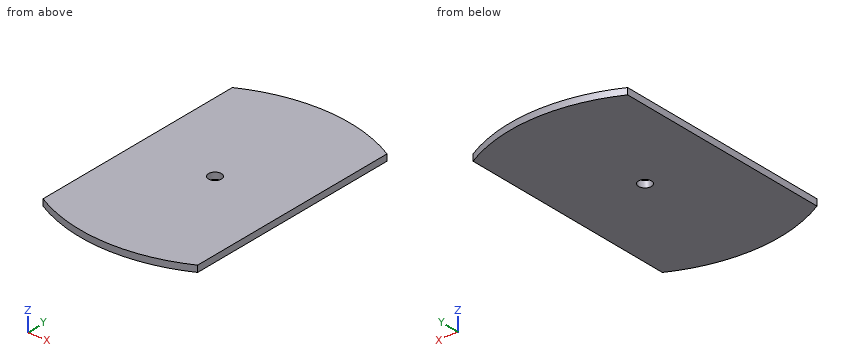
Autodesk Fusion 360 part; units mm, degrees
sketch "Esquisse1" plane through (0, 0, 0) normal (0, 0, 1) x (1, 0, 0)
  line L0 (60, -86) -> (-60, -86)
  line L1 (-60, -86) -> (-60, 86)
  line L2 (-60, 86) -> (60, 86)
  line L3 (60, 86) -> (60, -86)
  line L4 (60, -86) -> (-60, 86) construction
  line L5 (-60, -86) -> (60, 86) construction
  dimension "d1" = 120
  dimension "d2" = 172
sketch "Esquisse2" plane through (0, 0, 0) normal (0, 0, 1) x (1, 0, 0)
  line L0 (0, -86) -> (0, -101)
  line L1 (0, 86) -> (0, 101)
  line L2 (60, -86) -> (-60, -86)
  line L3 (-60, -86) -> (-60, -116)
  line L4 (-60, -116) -> (60, -116)
  line L5 (60, -116) -> (60, -86)
  line L6 (60, -86) -> (-60, -116) construction
  line L7 (-60, -86) -> (60, -116) construction
  line L8 (-60, 86) -> (60, 86)
  line L9 (60, 86) -> (60, 116)
  line L10 (60, 116) -> (-60, 116)
  line L11 (-60, 116) -> (-60, 86)
  line L12 (-60, 86) -> (60, 116) construction
  line L13 (60, 86) -> (-60, 116) construction
  arc A0 (60, 86) -> (-60, 86) centre (0, -26.5) ccw
  arc A1 (-60, -86) -> (60, -86) centre (0, 26.5) ccw
  point P0 (0, -101)
  point P1 (0, 101)
  dimension "d3" = 15
  dimension "d4" = 15
extrude "Extrusion1" add sketch "Esquisse1" sketch "Esquisse2" along normal blind 10 of sketch 2 contours L0 L2 A1 | L0 L2 A1 | L1 L8 A0 | L1 L8 A0
sketch "Esquisse3" plane through (0, 0, 10) normal (0, 0, 1) x (-1, 0, 0)
  line L0 (60, -86) -> (60, 86)
  arc A0 (60, 86) -> (-60, 86) centre (0, -26.5) ccw
  line L1 (-60, 86) -> (-60, -86)
  arc A1 (-60, -86) -> (60, -86) centre (0, 26.5) ccw
  line L2 (60, 86) -> (-60, 86)
  line L3 (60, -86) -> (-60, -86)
  line L4 (-60, 86) -> (-60, 70)
  line L5 (-60, 70) -> (-60, 48)
  line L6 (-60, 48) -> (-60, -48)
  line L7 (-60, -48) -> (-60, -70)
  line L8 (60, 86) -> (60, 70)
  line L9 (60, 70) -> (60, 48)
  line L10 (60, 48) -> (60, -48)
  line L11 (60, -48) -> (60, -70)
  line L12 (60, 70) -> (36, 70)
  line L13 (36, 70) -> (36, 48)
  line L14 (36, 48) -> (60, 48)
  line L15 (60, -70) -> (36, -70)
  line L16 (36, -70) -> (36, -48)
  line L17 (36, -48) -> (60, -48)
  line L18 (-60, -70) -> (-36, -70)
  line L19 (-36, -70) -> (-36, -48)
  line L20 (-36, -48) -> (-60, -48)
  line L21 (-60, 70) -> (-36, 70)
  line L22 (-36, 70) -> (-36, 48)
  line L23 (-60, 48) -> (-36, 48)
  dimension "d7" = 16
  dimension "d8" = 22
  dimension "d9" = 96
  dimension "d10" = 22
  dimension "d11" = 16
  dimension "d12" = 22
  dimension "d13" = 96
  dimension "d14" = 22
  dimension "d15" = 24
  dimension "d16" = 24
  dimension "d17" = 22
sketch "Esquisse4" plane through (0, 0, 10) normal (0, 0, 1) x (-1, 0, 0)
  line L0 (-60, -86) -> (-17, -86)
  line L1 (-17, -86) -> (17, -86)
  line L2 (17, -86) -> (17, -70)
  line L3 (17, -70) -> (-17, -70)
  line L4 (-17, -70) -> (-17, -86)
  dimension "d18" = 43
  dimension "d19" = 34
extrude "Extrusion2" cut sketch "Esquisse3" against normal blind 5
extrude "Extrusion3" cut sketch "Esquisse4" along normal blind 0 and the other way blind 25
sketch "Esquisse5" plane through (0, 0, 5) normal (0, 0, 1) x (-1, 0, 0)
  line L0 (17, -86) -> (-17, -86)
  line L1 (-17, -86) -> (-17, -70)
  line L2 (-17, -70) -> (17, -70)
  line L3 (17, -70) -> (17, -86)
  arc A0 (60, 86) -> (-60, 86) centre (0, -26.5) ccw
  line L4 (-60, 86) -> (-60, -86)
  arc A1 (-60, -86) -> (60, -86) centre (0, 26.5) ccw
  line L5 (60, -86) -> (60, 86)
  line L6 (-60, -86) -> (60, -86)
  line L7 (-60, 86) -> (60, 86)
  line L8 (-60, -86) -> (-60, -70)
  line L9 (-60, -70) -> (-60, -48)
  line L10 (-60, -48) -> (-60, 48)
  line L11 (-60, 48) -> (-60, 70)
  line L12 (-60, -70) -> (-36, -70)
  line L13 (-36, -70) -> (-36, -48)
  line L14 (-36, -48) -> (-60, -48)
  line L15 (-60, 70) -> (-36, 70)
  line L16 (-60, 48) -> (-36, 48)
  line L17 (-36, 48) -> (-36, 70)
  line L18 (60, -70) -> (36, -70)
  line L19 (36, -70) -> (36, -48)
  line L20 (36, -48) -> (60, -48)
  line L21 (60, 48) -> (36, 48)
  line L22 (36, 48) -> (36, 70)
  line L23 (36, 70) -> (60, 70)
  dimension "d27" = 16
  dimension "d28" = 22
  dimension "d29" = 96
  dimension "d30" = 22
  dimension "d31" = 24
  dimension "d32" = 24
sketch "Esquisse6" plane through (0, 0, 5) normal (0, 0, 1) x (-1, 0, 0)
  line L0 (27.5, -60) -> (-27.5, -60)
  line L1 (-27.5, -60) -> (-27.5, 7)
  line L2 (-27.5, 7) -> (27.5, 7)
  line L3 (27.5, 7) -> (27.5, -60)
  dimension "d34" = 55
  dimension "d35" = 67
sketch "Esquisse7" plane through (0, 0, 5) normal (0, 0, 1) x (-1, 0, 0)
  line L0 (27.5, 17) -> (-27.5, 17)
  line L1 (-27.5, 17) -> (-27.5, 83)
  line L2 (-27.5, 83) -> (27.5, 83)
  line L3 (27.5, 83) -> (27.5, 17)
  dimension "d38" = 55
  dimension "d39" = 66
extrude "Extrusion4" add sketch "Esquisse5" against normal blind 5 contours L0 L1 L2 L3 L6
sketch "Esquisse8" plane through (0, 0, 5) normal (0, 0, 1) x (-1, 0, 0)
  arc A0 (60, 86) -> (-60, 86) centre (0, -26.5) ccw
  line L0 (-60, 86) -> (-60, -86)
  arc A1 (-60, -86) -> (60, -86) centre (0, 26.5) ccw
  line L1 (60, -86) -> (60, 86)
  circle A2 centre (0, 0) radius 5
  dimension "d42" = 10
extrude "Extrusion5" cut sketch "Esquisse8" against normal blind 5 contours A2
sketch "Esquisse9" plane through (0, 0, 5) normal (0, 0, 1) x (-1, 0, 0)
  circle A0 centre (0, 0) radius 5
  arc A1 (60, 86) -> (-60, 86) centre (0, -26.5) ccw
  line L0 (-60, 86) -> (-60, -86)
  arc A2 (-60, -86) -> (60, -86) centre (0, 26.5) ccw
  line L1 (60, -86) -> (60, 86)
  line L2 (60, 86) -> (-60, 86)
  line L3 (60, -86) -> (-60, -86)
Build history of the part. All positions in model axes, mm. Coordinates: 2 decimals unless noted, no trailing zeros. Write each loop counter-clockwise with the first axis right and the second up, starting at its lowest first coordinate (ties: lowest second). Pieces come first, ordered by that corner, then holes.
(1) Cut at A-A on y = 0. List the corners of the cut face in (x, z), and give its area (3 significant figures).
(2) Cut at D-D on x = -47. List the corners of the cut face in (y, z), and give its area (3 significant figures).
(3) Cut at C-C on z = 3.85. List the corners of the cut face in (x, y), and give its area (3 significant figures).
(4) Drill centre lines: line 1 (Y direction, x = 0, z = 3); line 2 (X direction, y = 0, z = 2.05); line 3 (Y direction, x = -24.5, z = 3.3). Where is each one in solid material? Low to high.
(5) Cut at B-B on x = 0. List the corners of the cut face in (y, z), and give its area (3 significant figures).
(6) Pin check, flat tip, straight feed: pin 1 Ø3 at (x, z) = (-6.5, 1.5) entering from +Y. Stop position of the tip, or through.
Working result:
1. outline: (-60, 0) - (-5, 0) - (-5, 5) - (-60, 5) - close; (5, 0) - (60, 0) - (60, 5) - (5, 5) - close
1. area: 550 mm2
2. outline: (-92.02, 0) - (92.02, 0) - (92.02, 5) - (-92.02, 5) - close
2. area: 920 mm2
3. outline: (-60, -86) arc R127.5 ccw to (60, -86) - (60, 86) arc R127.5 ccw to (-60, 86) - close; hole circle Ø10 at (0, 0)
3. area: 23,000 mm2
4. line 1: y = -101 to -5, 5 to 101
4. line 2: x = -60 to -5, 5 to 60
4. line 3: y = -98.62 to 98.62
5. outline: (-101, 0) - (-5, 0) - (-5, 5) - (-101, 5) - close; (5, 0) - (101, 0) - (101, 5) - (5, 5) - close
5. area: 960 mm2
6. pin 1: stops at y = 100.9
